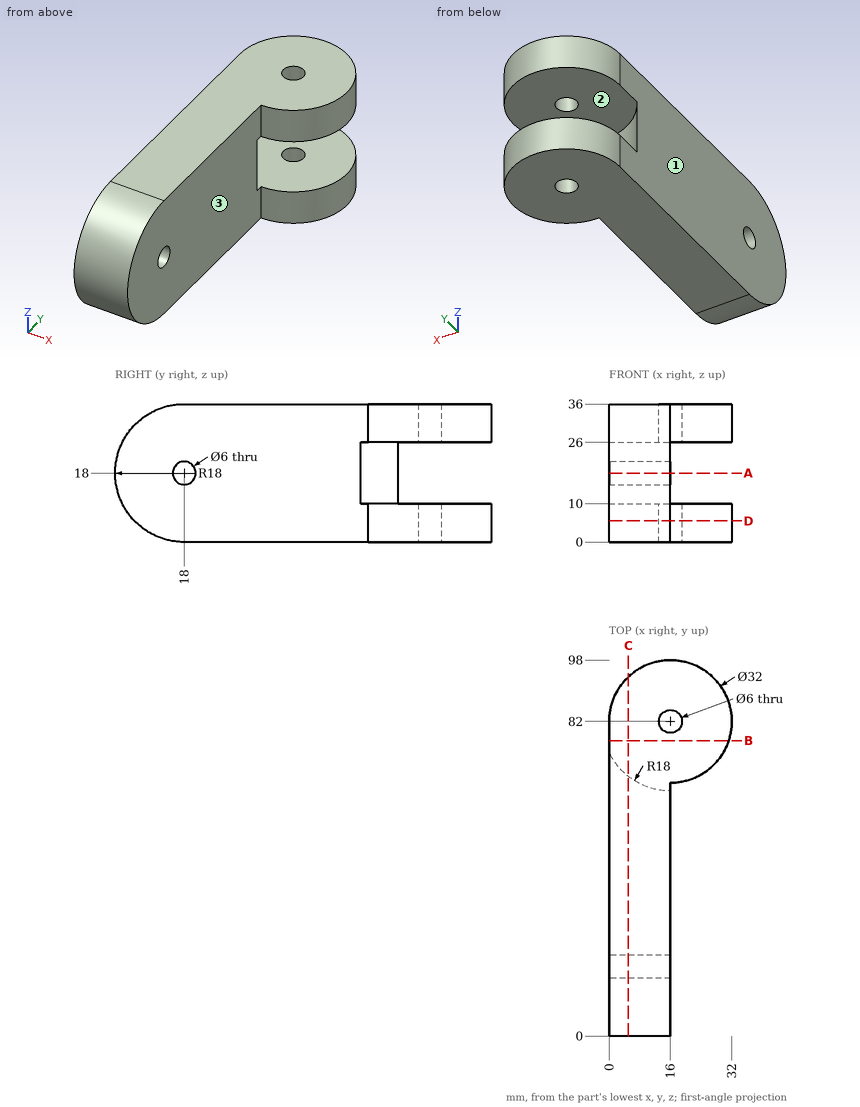
Print and shaded views of the part. All mm, measured from the part's lowest x, y and z. A direction names the side the tool comes from. Round coordinates to 2 decimals unless told otherwise and drop trailing zeros. Write each loop counter-clockwise with the first axis right and the second up, starting at its lowest first coordinate (ties: lowest second). Pieces come first, ordered by that corner, then holes. Notation, with made-up numbers: (-33.5, -0.75) -> (25.5, -0.75) arc R30 cw to (25.5, 25.25) -> close; hole circle Ø10 at (-18.5, -1.5). An arc over 180 degrees is marked (long way). Answer in a Markdown table with one row per item. Add a question column.
Item 1: Drill centre lines: line 1 (Z direction, x = 22, y = 68); line 2 (X direction, y = 52.5, z = 5); line 3 (Y direction, x = 3.5, z = 18). Where is each one in solid material? Low to high. Write a range as from..to.
Item 2: Drop flat-ended pins along their axis: pin 1 Ø8 at (x, z) = (18.5, 17) entering from +Y; pin 2 Ø1 at (y, z) = (17.5, 9) entering from +X; pin 3 Ø1.5 at (x, z) = (22, 9.5) entering from +Y. Give the stop position or say it passes through.
Item 3: Which spindle directions (+Z, -Z, +X, -X, +Y, -Y) get a long thin tool onto all of the face, cutting with end or side? Do the marked faces 1, 2 and 3. Say none if no direction does.
Item 4: Saw through at A-A, the plane z = 18. Write the cut outline in (x, y).
Item 5: Saw through at C-C, the plane x = 5. Write the cut outline in (y, z).
Item 6: Saw through at D-D, the plane z = 5.5. Write the cut outline in (x, y).
Item 7: Saw through at B-B, the plane y = 77. Write the cut outline in (x, z), then the cut area to 3 significant figures.
Findings below:
| question | item | result |
|---|---|---|
| 1 | line 1 | z = 0..10, 26..36 |
| 1 | line 2 | x = 0..16 |
| 1 | line 3 | y = 0..15, 21..69.05 |
| 2 | pin 1 | stops at y = 64.06 |
| 2 | pin 2 | stops at x = 16 |
| 2 | pin 3 | stops at y = 97.11 |
| 3 | face 1 | +Z, -Z, -X, +Y, -Y |
| 3 | face 2 | +X, +Y |
| 3 | face 3 | +Z, -Z, +X, -Y |
| 4 | outline | (0, 0) -> (16, 0) -> (16, 15) -> (0, 15) -> close; (0, 21) -> (16, 21) -> (16, 64) arc R18 cw to (0, 73.75) -> close |
| 5 | outline | (18, 0) -> (93.62, 0) -> (93.62, 10) -> (67.75, 10) -> (67.75, 26) -> (93.62, 26) -> (93.62, 36) -> (18, 36) arc R18 ccw to start; hole circle Ø6 at (18, 18) |
| 6 | outline | (0, 5.05) -> (16, 5.05) -> (16, 66) arc R16 ccw (long way) to (0, 82) -> close; hole circle Ø6 at (16, 82) |
| 7 | outline | (0, 0) -> (31.2, 0) -> (31.2, 10) -> (0, 10) -> close; (0, 26) -> (31.2, 26) -> (31.2, 36) -> (0, 36) -> close |
| 7 | area | 624 mm^2 |
